Autodesk Fusion 360 part; units mm, degrees
sketch "Sketch2" plane through (0, 0, 0) normal (0, 0, 1) x (1, 0, 0)
  line L0 (-18, 55) -> (7, 55)
  line L1 (7, 55) -> (71, 55)
  line L2 (71, 55) -> (96, 55)
  line L3 (96, -9) -> (96, 23)
  line L4 (96, 23) -> (96, 55)
  line L5 (96, -9) -> (71, -9)
  line L6 (71, -9) -> (58, -9)
  line L7 (58, -9) -> (20, -9)
  line L8 (20, -9) -> (7, -9)
  line L9 (7, -9) -> (-18, -9)
  line L10 (71, -9) -> (71, 55)
  line L11 (58, -9) -> (58, 42)
  line L12 (58, 42) -> (20, 42)
  line L13 (20, 42) -> (20, -9)
  line L14 (7, -9) -> (7, 55)
  line L15 (-18, -9) -> (-18, 55)
  circle A0 centre (96, 23) radius 32
  circle A1 centre (-18, 23) radius 32
  circle A2 centre (-18, 23) radius 11
  circle A3 centre (96, 23) radius 11
  dimension "d7" = 25
  dimension "d8" = 64
  dimension "d9" = 25
  dimension "d13" = 32
  dimension "d14" = 25
  dimension "d15" = 13
  dimension "d16" = 38
  dimension "d17" = 13
  dimension "d18" = 25
  dimension "d20" = 51
  dimension "d21" = 38
  dimension "d23" = 22
  dimension "d24" = 22
extrude "Extrude1" add sketch "Sketch2" along normal blind 19 contours L14 L15 A1 A2 | L15 A1 A2 | L0 L14 A1 | L9 L14 A1 | L2 L10 A0 | L3 L4 A0 A3 | L3 L4 L10 A0 A3 | L5 L10 A0 makes body 1 at (85.8333, -1.5088, 19) makes body 2 at (-7.8333, -1.5088, 0)
extrude "Extrude2" add sketch "Sketch2" along normal blind 64 contours L1 L6 L8 L10 L11 L12 L13 L14 A0 A1 | L14 A1 | L10 A0 bodies 1 2
ref_plane "WorkPlane1" through (39, -9, 0) normal (0, -0.7071, 0.7071) x (-1, 0, 0)
extrude "Extrude3" add sketch "Sketch2" along normal blind 13 contours L7 L11 L12 L13 start surface through (39, -9, 0) normal (0, -0.707107, 0.707107) bodies 1
Geometry check sheet. Reference: the model listing, model coordinates, mm. A direction names the side the tool comes from. Round coordinates to 2 decimals unless told otherwise and drop trailing zeros. Loops run counter-clockwise (first coordinate to the right, second up) from the corner with the lowest first, then second, coordinate; pieces in that order, holes last. Notation, with made-up numbers: M 14,-28.75 L 32,-28.75 A13 ccw 32,-7.75 Z; hole C 75,44.25 d9. An arc over 180 degrees is marked long. Return JSON: item names as keys, results as strings. Group by question number.
(1) Set-up check for faces 1 (the face through (39, 17, 30)), 2 (the face through (-28, 31, 19)), 3 (the face through (38, 55, 24)), 4 (the face through (39, 17, 17)), 5 (the face through (105, 31, 19)): record each of +Z, -Z, +X, -X, +Y, -Y from which the full face is reachable in a straight line by a thin tool's end or side.
(2) Section check C-C, the plane y = 4. Enter the section's corners in (x, z).
(3) Section check A-A, the plane y = 23. Enter the section's corners in (x, z).
(4) Section check B-B, the plane z = 54. Enter the section's corners in (x, y).
(5) Scan lines: line 1 along X through (y, z) = (23, 6.25); line 2 along Y through (x, z) = (96, 7.25); line 3 along Z through (x, y) = (114, -1). Record each from-to range of solid material in increasing order. Write a range as [from, to].
(6) Go/stop test with flat-tipped pins: pin 1 (6 mm diameter, centred on x = 41.5, z = 46, fed in from -Y); pin 2 (4 mm diameter, centred on x = -21.5, z = 6.5, fed in from -Y); pin 3 (18.5 mm diameter, centred on y = 12, z = 8, fed in from +X). Record where each tip stops, or that it passes through.
(7) Mould release check, pull along Y, two halves, no side actions. Record for faces 6 (the face through (127.992, 23.704, 9.367)), 7 (the face through (-20.38, 33.74, 9.37)), 8 (the face through (39, 42, 8)), 9 (the face through (85, 23, 9)): pulls with the +Y half, pulls with the -Y half, needs draft (parallel to the pull), parting line crosses it, or undercut.
(8) Section check D-D, the plane z = 25. Enter the section's corners in (x, y).
Data:
{
 "1": {"face 1": "+Z, -Y", "face 2": "+Z, -X, +Y, -Y", "face 3": "+Z, -Z, +X, -X, +Y", "face 4": "-Z, -Y", "face 5": "+Z, +X, +Y, -Y"},
 "2": {"outline": "M -43.75,0 L 20,0 L 20,17 L 58,17 L 58,0 L 121.75,0 L 121.75,19 L 71,19 L 71,64 L 58,64 L 58,30 L 20,30 L 20,64 L 7,64 L 7,19 L -43.75,19 Z"},
 "3": {"outline": "M -50,0 L -29,0 L -29,19 L -50,19 Z; M -7,0 L 20,0 L 20,17 L 58,17 L 58,0 L 85,0 L 85,19 L 71,19 L 71,64 L 58,64 L 58,30 L 20,30 L 20,64 L 7,64 L 7,19 L -7,19 Z; M 107,0 L 128,0 L 128,19 L 107,19 Z"},
 "4": {"outline": "M 7,-9 L 20,-9 L 20,42 L 58,42 L 58,-9 L 71,-9 L 71,55 L 7,55 Z"},
 "5": {"line 1": "[-50, -29], [-7, 20], [58, 85], [107, 128]", "line 2": "[-9, 12], [34, 55]", "line 3": "[0, 19]"},
 "6": {"pin 1": "y = 42", "pin 2": "y = -8.96", "pin 3": "x = 127.95"},
 "7": {"face 6": "parting line crosses it", "face 7": "undercut", "face 8": "pulls with the -Y half", "face 9": "undercut"},
 "8": {"outline": "M 7,-9 L 71,-9 L 71,55 L 7,55 Z"}
}
